Model file for the job. Use its own axes, mm. A direction names the side the tool comes from. Round coordinates to 2 decimals unless told otherwise and drop trailing zeros. Loops run counter-clockwise (first coordinate to the right, second up) from the corner with the lowest first, then second, coordinate; pieces in that order, holes last. Notation, with made-up numbers: (88, 5) -> (106, 5) arc R16 ccw to (106, 24) -> close; hole circle Ø5 at (13.25, 73.5). An arc over 180 degrees is marked (long way). Use a Markdown table: item, result.
from build123d import *

# Parameters (mm, degrees)
SKETCH1_R           = 5
SKETCH1_R_2         = 2.83
BOSS_EXTRUDE1_DEPTH = 4


with BuildPart() as part:
    # Sketch1 → Boss-Extrude1 (new body)
    with BuildSketch(Plane.XY):
        Polygon((47, 30), (54.5, 30), (54.5, 25.25), (62.5, 25.25), (62.5, 17.25), (54.5, 17.25), (54.5, 12.5), (47, 12.5), (47, -30), (-81, -30), (-81, 30), align=None)
        with Locations((-36, 0)):
            Circle(SKETCH1_R, mode=Mode.SUBTRACT)
        with Locations((14, -24)):
            Circle(SKETCH1_R_2, mode=Mode.SUBTRACT)
    extrude(amount=BOSS_EXTRUDE1_DEPTH)


solid = part.part
Q1. Pull direction Y, two halves, no side cores. Call faces 4 (the face through (-41, 0, 2)), 5 (the face through (-12, 30, 2)), 6 (the face through (59, 17.25, 2)): released by +Y, released by -Y, zero draft, split by the parting line, or undercut.
Results list:
| item | result |
|---|---|
| face 4 | undercut |
| face 5 | released by +Y |
| face 6 | released by -Y |
Q2. Drill centre lines: L1, parallel to Y at x = -36, z = 1; L2, parallel to Y at x = 52.5, z = 2.7; L3, parallel to X at y = -9, z = 0.8. Where is each one in solid material? Low to high. Write a range as from..to.
Results list:
| item | result |
|---|---|
| L1 | y = -30..-5, 5..30 |
| L2 | y = 12.5..30 |
| L3 | x = -81..47 |
Q3. Band-saw the part on A-A, the plane x = 14. Give the cut face in (y, z), plus the area to 3 significant figures.
Results list:
| item | result |
|---|---|
| outline | (-30, 0) -> (-26.83, 0) -> (-26.83, 4) -> (-30, 4) -> close; (-21.17, 0) -> (30, 0) -> (30, 4) -> (-21.17, 4) -> close |
| area | 217 mm² |
Q4. Band-saw the part on B-B, the plane y = -24. Give the cut face in (x, z).
Results list:
| item | result |
|---|---|
| outline | (-81, 0) -> (11.17, 0) -> (11.17, 4) -> (-81, 4) -> close; (16.83, 0) -> (47, 0) -> (47, 4) -> (16.83, 4) -> close |
Q5. Band-saw the part on D-D, the plane y = -17.5. Give the cut face in (x, z).
Results list:
| item | result |
|---|---|
| outline | (-81, 0) -> (47, 0) -> (47, 4) -> (-81, 4) -> close |
Q6. Band-saw the part on C-C, the plane z = 0.85. Give the cut face in (x, y), plus the area to 3 significant figures.
Results list:
| item | result |
|---|---|
| outline | (-81, -30) -> (47, -30) -> (47, 12.5) -> (54.5, 12.5) -> (54.5, 17.25) -> (62.5, 17.25) -> (62.5, 25.25) -> (54.5, 25.25) -> (54.5, 30) -> (-81, 30) -> close; hole circle Ø10 at (-36, 0); hole circle Ø5.66 at (14, -24) |
| area | 7,770 mm² |
Q7. Tool access for faces 1 (the face through (54.5, 28, 2)), 2 (the face through (51, 12.5, 2)), 3 (the face through (-81, 0, 2)): list every direction of +Z, -Z, +X, -X, +Y, -Y with a clear straight run to the whole face (end or side of a thin tool).
Results list:
| item | result |
|---|---|
| face 1 | +Z, -Z, +X, +Y |
| face 2 | +Z, -Z, +X, -Y |
| face 3 | +Z, -Z, -X, +Y, -Y |
Q8. Flat gauge pins, fed straight in: pin 1 (8 mm diameter, centred on x = -36, y = 0, fed in from +Z); pin 2 (1.2 mm diameter, centred on x = 60.5, z = 2.5, fed in from +Y); pin 3 (1.2 mm diameter, centred on x = 58.5, z = 1.5, fed in from -Y); pin 4 (1 mm diameter, centred on y = -3.5, z = 1.5, fed in from +X). Where does each tip first touch, or does it go through?
Results list:
| item | result |
|---|---|
| pin 1 | passes through |
| pin 2 | stops at y = 25.25 |
| pin 3 | stops at y = 17.25 |
| pin 4 | stops at x = 47 |
